Part model, mm, in its own coordinate system. A direction names the side the tool comes from. Coordinates: 2 decimals unless noted, no trailing zeros. Loops run counter-clockwise (first coordinate to the right, second up) from the corner with the lowest first, then second, coordinate; pieces in that order, holes last. Notation, with made-up numbers: M 43,-38 L 51,-38 A10 cw 51,-24 Z; hole C 54,35 d7. An arc over 180 degrees is marked long. Answer as CSV lines item,"result". Start each with the question number.
from build123d import *

# Parameters (mm, degrees)
SKETCH1_R               = 17.018
SKETCH1_R_2             = 3.683
SKETCH1_W               = 14.986
SKETCH1_H               = 13.843
BOSS_EXTRUDE2_DEPTH     = 22.098
DRAFT2_ANGLE            = -5
BOSS_EXTRUDE3_DEPTH     = 5.334
CUT_EXTRUDE1_DEPTH      = 97.762405579
CUT_EXTRUDE1_DEPTH_BACK = 97.762405579
CUT_EXTRUDE2_DEPTH      = 97.762405579
CUT_EXTRUDE2_DEPTH_BACK = 97.762405579
BOSS_EXTRUDE4_DEPTH     = 10.668


with BuildPart() as part:
    # Sketch1 → Boss-Extrude2 (new body)
    with BuildSketch(Plane(origin=(0, 0, 0), x_dir=(1, 0, 0), z_dir=(0, 1, 0))):
        with BuildLine():
            Line((-50.551365501, 53.976983945), (-30.231365501, 53.976983945))
            Line((-30.231365501, 53.976983945), (-30.231365501, 36.322144789))
            Line((-30.231365501, 36.322144789), (-19.670165688, 32.890602954))
            ThreePointArc((-19.670165688, 32.890602954), (-15.733165688, 30.030205021), (-14.229365501, 25.401983945))
            Line((-14.229365501, 25.401983945), (-14.229365501, -38.098016055))
            ThreePointArc((-14.229365501, -38.098016055), (-15.733165688, -42.726237132), (-19.670165688, -45.586635064))
            Line((-19.670165688, -45.586635064), (-30.231365501, -49.0181769))
            Line((-30.231365501, -49.0181769), (-30.231365501, -66.673016055))
            Line((-30.231365501, -66.673016055), (-50.551365501, -66.673016055))
            Line((-50.551365501, -66.673016055), (-50.551365501, -49.0181769))
            Line((-50.551365501, -49.0181769), (-61.112565315, -45.586635064))
            ThreePointArc((-61.112565315, -45.586635064), (-65.049565315, -42.726237132), (-66.553365501, -38.098016055))
            Line((-66.553365501, -38.098016055), (-66.553365501, 25.401983945))
            ThreePointArc((-66.553365501, 25.401983945), (-65.049565315, 30.030205021), (-61.112565315, 32.890602954))
            Line((-61.112565315, 32.890602954), (-50.551365501, 36.322144789))
            Line((-50.551365501, 36.322144789), (-50.551365501, 53.976983945))
        make_face()
        with Locations(Location((-40.391365501, -6.348016055, 0), (0, 0, 270))):
            Circle(SKETCH1_R, mode=Mode.SUBTRACT)
        with Locations(Location((-22.103365501, 25.401983945, 0), (0, 0, 270))):
            Circle(SKETCH1_R_2, mode=Mode.SUBTRACT)
        with Locations(Location((-58.679365501, 25.401983945, 0), (0, 0, 270))):
            Circle(SKETCH1_R_2, mode=Mode.SUBTRACT)
        with Locations(Location((-58.679365501, -38.098016055, 0), (0, 0, 270))):
            Circle(SKETCH1_R_2, mode=Mode.SUBTRACT)
        with Locations(Location((-22.103365501, -38.098016055, 0), (0, 0, 270))):
            Circle(SKETCH1_R_2, mode=Mode.SUBTRACT)
        with Locations((-40.391365501, 44.388483945)):
            Rectangle(SKETCH1_W, SKETCH1_H, mode=Mode.SUBTRACT)
        with Locations((-40.391365501, -57.084516055)):
            Rectangle(SKETCH1_W, SKETCH1_H, mode=Mode.SUBTRACT)
    extrude(amount=BOSS_EXTRUDE2_DEPTH)

    # Draft2
    draft2_faces = [part.faces().sort_by_distance(p)[0] for p in [
        (-55.831965408, 11.049, -34.606373872),
        (-65.049565315, 11.049, -30.030205021),
        (-66.553365501, 11.049, 6.348016055),
        (-65.049565315, 11.049, 42.726237132),
        (-55.831965408, 11.049, 47.302405982),
        (-15.733165688, 11.049, 42.726237132),
        (-24.950765594, 11.049, 47.302405982),
        (-24.950765594, 11.049, -34.606373872),
        (-15.733165688, 11.049, -30.030205021),
        (-14.229365501, 11.049, 6.348016055),
    ]]
    draft(draft2_faces, Plane(origin=(0, 0, 0), x_dir=(0, 0, -1), z_dir=(0, -1, 0)), DRAFT2_ANGLE)

    # Sketch1_4 → Boss-Extrude3 (add)
    with BuildSketch(Plane(origin=(0, 0, 0), x_dir=(1, 0, 0), z_dir=(0, 1, 0))):
        with BuildLine():
            Line((-40.391365501, -54.735016055), (-40.391365501, -50.163016055))
            Line((-40.391365501, -50.163016055), (-47.884365501, -50.163016055))
            Line((-47.884365501, -50.163016055), (-47.884365501, -64.006016055))
            Line((-47.884365501, -64.006016055), (-40.391365501, -64.006016055))
            Line((-40.391365501, -64.006016055), (-40.391365501, -62.101016055))
            ThreePointArc((-40.391365501, -62.101016055), (-44.074365501, -58.418016055), (-40.391365501, -54.735016055))
        make_face()
        with BuildLine():
            Line((-32.898365501, -50.163016055), (-40.391365501, -50.163016055))
            Line((-40.391365501, -50.163016055), (-40.391365501, -54.735016055))
            ThreePointArc((-40.391365501, -54.735016055), (-37.787091226, -55.81374178), (-36.708365501, -58.418016055))
            ThreePointArc((-36.708365501, -58.418016055), (-37.787091226, -61.02229033), (-40.391365501, -62.101016055))
            Line((-40.391365501, -62.101016055), (-40.391365501, -64.006016055))
            Line((-40.391365501, -64.006016055), (-32.898365501, -64.006016055))
            Line((-32.898365501, -64.006016055), (-32.898365501, -50.163016055))
        make_face()
        with BuildLine():
            Line((-40.391365501, 49.404983945), (-40.391365501, 51.309983945))
            Line((-40.391365501, 51.309983945), (-47.884365501, 51.309983945))
            Line((-47.884365501, 51.309983945), (-47.884365501, 37.466983945))
            Line((-47.884365501, 37.466983945), (-40.391365501, 37.466983945))
            Line((-40.391365501, 37.466983945), (-40.391365501, 42.038983945))
            ThreePointArc((-40.391365501, 42.038983945), (-44.074365501, 45.721983945), (-40.391365501, 49.404983945))
        make_face()
        with BuildLine():
            Line((-32.898365501, 51.309983945), (-40.391365501, 51.309983945))
            Line((-40.391365501, 51.309983945), (-40.391365501, 49.404983945))
            ThreePointArc((-40.391365501, 49.404983945), (-37.787091226, 48.32625822), (-36.708365501, 45.721983945))
            ThreePointArc((-36.708365501, 45.721983945), (-37.787091226, 43.11770967), (-40.391365501, 42.038983945))
            Line((-40.391365501, 42.038983945), (-40.391365501, 37.466983945))
            Line((-40.391365501, 37.466983945), (-32.898365501, 37.466983945))
            Line((-32.898365501, 37.466983945), (-32.898365501, 51.309983945))
        make_face()
    extrude(amount=BOSS_EXTRUDE3_DEPTH)

    # Sketch2 → Cut-Extrude1 (cut, two sides: drawn at the far end of the back side and taken through both)
    with BuildSketch(Plane(origin=(0, 0, 0), x_dir=(0, 0, -1), z_dir=(1, 0, 0)).offset(-CUT_EXTRUDE1_DEPTH_BACK)):
        Polygon((-66.673016055, 4.318), (-66.673016055, 22.098), (-48.893016055, 22.098), align=None)
        Polygon((36.196983945, 22.098), (53.976983945, 22.098), (53.976983945, 4.318), align=None)
    extrude(amount=CUT_EXTRUDE1_DEPTH + CUT_EXTRUDE1_DEPTH_BACK, mode=Mode.SUBTRACT)

    # Sketch3 → Cut-Extrude2 (cut, two sides: drawn at the far end of the back side and taken through both)
    with BuildSketch(Plane.XY.offset(-CUT_EXTRUDE2_DEPTH_BACK)):
        Polygon((-40.391365501, 22.098), (-64.620041015, 22.098), (-64.99966368, 17.758893082), align=None)
        Polygon((-16.162689988, 22.098), (-40.391365501, 22.098), (-15.783067323, 17.758893082), align=None)
    extrude(amount=CUT_EXTRUDE2_DEPTH + CUT_EXTRUDE2_DEPTH_BACK, mode=Mode.SUBTRACT)

    # Sketch1_5 → Boss-Extrude4 (add)
    with BuildSketch(Plane(origin=(0, 0, 0), x_dir=(1, 0, 0), z_dir=(0, 1, 0))):
        with BuildLine():
            ThreePointArc((-23.373365501, -6.348016055), (-28.357822299, 5.685527147), (-40.391365501, 10.669983945))
            Line((-40.391365501, 10.669983945), (-40.391365501, 7.240983945))
            ThreePointArc((-40.391365501, 7.240983945), (-30.782491452, 3.260857994), (-26.802365501, -6.348016055))
            ThreePointArc((-26.802365501, -6.348016055), (-30.782491452, -15.956890105), (-40.391365501, -19.937016055))
            Line((-40.391365501, -19.937016055), (-40.391365501, -23.366016055))
            ThreePointArc((-40.391365501, -23.366016055), (-28.357822299, -18.381559257), (-23.373365501, -6.348016055))
        make_face()
        with BuildLine():
            Line((-40.391365501, 7.240983945), (-40.391365501, 10.669983945))
            ThreePointArc((-40.391365501, 10.669983945), (-57.409365501, -6.348016055), (-40.391365501, -23.366016055))
            Line((-40.391365501, -23.366016055), (-40.391365501, -19.937016055))
            ThreePointArc((-40.391365501, -19.937016055), (-53.980365501, -6.348016055), (-40.391365501, 7.240983945))
        make_face()
    extrude(amount=BOSS_EXTRUDE4_DEPTH)


solid = part.part
Q1. Slice it at C-C, the plane y = 14. State how many separate pieces and enclosed holes the cut face has, and give its area (3 significant figures).
Q2. Tool access for faces 5 (the face through (-32.898, 11, -43)), 6 (the face through (-15, 8.8, 5.9)), 7 (the face through (-50.551, 8, 55)): list every direction of +Z, -Z, +X, -X, +Y, -Y with a clear straight run to the whole face (end or side of a thin tool).
Q3. Two-plate mould, pull along X, no slides. Class faces 1 (the face through (-30.231, 8, 55)), 2 (the face through (-40, 2, 66.673)), 3 (the face through (-55.028, 9.689, 37.619)), 4 (the face through (-47.884, 11, -43)): +X half, -X half, draft (parallel to the pull), parting line (faces both ways), or undercut.
Q4. Slice it at B-B, the plane z = 16.5. Write the cut outline in (x, y).
Q5. Flat gauge pins, fed straight in: P1, Ø2, axis at x = -43, z = -36, coming from the +Y side; P2, Ø1, axis at x = -53, z = 38.5, coming from the -Y side; P3, Ø10, axis at y = 7, z = 0, coming from the -X side; P4, Ø12, axis at x = -22.1, z = -25.4, coming from the +Y side. Where does each tip first touch, or does it go through?
Q6. Slice it at A-A, the plane x = -52. Write the cut outline in (y, z).
Q7. Slice it at D-D, the plane z = -15.5. Write the cut outline in (x, y).
Q8. Wall check: L1, parallel to X at y = 9.5, z = 59; L2, parallel to Z at x = -56, y = 12; L3, parallel to Z at x = -25, y = 10. Give the ranges that are in metal, low to high.
Solved:
1,separate pieces,"1"
1,enclosed holes,"5"
1,area,"3,060 mm2"
2,face 5,"+Y"
2,face 6,"+Z, -Z, +X, +Y"
2,face 7,"+Z, -X, +Y"
3,face 1,"+X half"
3,face 2,"draft"
3,face 3,"undercut"
3,face 4,"undercut"
4,outline,"M -66.55,0 L -49.42,0 L -49.42,10.67 L -54.05,10.67 L -54.05,19.69 L -65,17.76 Z; M -31.36,0 L -14.23,0 L -15.78,17.76 L -26.73,19.69 L -26.73,10.67 L -31.36,10.67 Z"
5,P1,"stops at y = 21.81"
5,P2,"stops at y = 0"
5,P3,"stops at x = -66.38"
5,P4,"stops at y = 19.93"
6,outline,"M 0,-35.85 L 20.05,-34.01 L 20.05,-6.1 L 10.67,-6.1 L 10.67,-0.72 L 0,-0.72 Z; M 0,13.41 L 10.67,13.41 L 10.67,18.79 L 20.05,18.79 L 20.05,46.7 L 0,48.55 Z"
7,outline,"M -66.55,0 L -14.23,0 L -15.78,17.76 L -40.39,22.1 L -65,17.76 Z"
8,L1,"x = -50.55 to -47.88, -32.9 to -30.23"
8,L2,"z = -33.45 to -27.93, -22.88 to -0.43, 13.13 to 35.57, 40.62 to 46.14"
8,L3,"z = -33.7 to -27.68, -23.13 to 35.82, 40.37 to 46.4"
